from build123d import *

# Parameters (mm, degrees)
BOSS_EXTRUDE1_DEPTH       = 5.588
F_6_32_TAPPED_HOLE1_D     = 2.7051
F_6_32_TAPPED_HOLE1_DEPTH = 0.508
CUT_EXTRUDE1_REACH        = 12.16
SKETCH6_R                 = 2.159
CUT_EXTRUDE2_DEPTH        = 6.588
BOSS_EXTRUDE3_DEPTH       = 1.016
SKETCH20_W                = 9.144
SKETCH20_H                = 2.56692539
CUT_EXTRUDE3_DEPTH        = 8.382
SKETCH22_W                = 9.144
SKETCH22_H                = 8.382
BOSS_EXTRUDE4_DEPTH       = 0.508
SKETCH24_W                = 9.144
SKETCH24_H                = 8.382
BOSS_EXTRUDE5_DEPTH       = 0.508


with BuildPart() as part:
    # Sketch1 → Boss-Extrude1 (new body)
    with BuildSketch(Plane.XY):
        Polygon((-3.353873239, 7.634688699), (-3.353873239, -2.271311301), (6.806126761, -2.271311301), (6.806126761, 7.634688699), (6.298126761, 7.634688699), (6.298126761, -0.747311301), (-2.845873239, -0.747311301), (-2.845873239, 7.634688699), align=None)
    extrude(amount=BOSS_EXTRUDE1_DEPTH)

    # #6-32 Tapped Hole1
    with Locations(Plane.ZY.offset(3.353873239)):
        with Locations((2.794, 4.840688699)):
            Hole(F_6_32_TAPPED_HOLE1_D / 2, depth=F_6_32_TAPPED_HOLE1_DEPTH)

    # Sketch6 → Cut-Extrude1 (cut, up to next)
    with BuildSketch(Plane(origin=(6.806126761, 0, 0), x_dir=(0, 0, -1), z_dir=(1, 0, 0)), mode=Mode.PRIVATE) as cut_extrude1_sk1:
        with Locations((-2.794, 4.840688699)):
            Circle(SKETCH6_R)
    cut_extrude1_tool1 = extrude(cut_extrude1_sk1.sketch, amount=-CUT_EXTRUDE1_REACH, mode=Mode.PRIVATE) & part.part
    add(cut_extrude1_tool1.solids().sort_by_distance((6.806127, 4.840689, 2.794))[0], mode=Mode.SUBTRACT)

    # Sketch16 → Cut-Extrude2 (cut, through all)
    with BuildSketch(Plane(origin=(0, 0, 0), x_dir=(-1, 0, 0), z_dir=(0, 0, -1))):
        with BuildLine():
            Line((3.353873239, -2.271311301), (-6.806126761, -2.271311301))
            ThreePointArc((-6.806126761, -2.271311301), (-1.726126761, -1.350821544), (3.353873239, -2.271311301))
        make_face()
    extrude(amount=-CUT_EXTRUDE2_DEPTH, mode=Mode.SUBTRACT)

    # Sketch19 → Boss-Extrude3 (add)
    with BuildSketch(Plane.XY.offset(5.588)):
        with BuildLine():
            Line((6.806126761, 7.634688699), (6.298126761, 7.634688699))
            Line((6.298126761, 7.634688699), (-2.845873239, 7.634688699))
            Line((-2.845873239, 7.634688699), (-3.353873239, 7.634688699))
            Line((-3.353873239, 7.634688699), (-3.353873239, -2.271311301))
            ThreePointArc((-3.353873239, -2.271311301), (1.726126761, -1.350821544), (6.806126761, -2.271311301))
            Line((6.806126761, -2.271311301), (6.806126761, 7.634688699))
        make_face()
    extrude(amount=BOSS_EXTRUDE3_DEPTH)

    # Sketch20 → Cut-Extrude3 (cut)
    with BuildSketch(Plane(origin=(0, 7.634688699, 0), x_dir=(1, 0, 0), z_dir=(0, 1, 0))):
        with Locations((1.726126761, -6.871462695)):
            Rectangle(SKETCH20_W, SKETCH20_H)
    extrude(amount=-CUT_EXTRUDE3_DEPTH, mode=Mode.SUBTRACT)

    # Sketch22 → Boss-Extrude4 (add)
    with BuildSketch(Plane.XY.offset(6.604)):
        with Locations((1.726126761, 3.443688699)):
            Rectangle(SKETCH22_W, SKETCH22_H)
    extrude(amount=-BOSS_EXTRUDE4_DEPTH)

    # Sketch24 → Boss-Extrude5 (add)
    with BuildSketch(Plane(origin=(0, 0, 0), x_dir=(-1, 0, 0), z_dir=(0, 0, -1))):
        with Locations((-1.726126761, 3.443688699)):
            Rectangle(SKETCH24_W, SKETCH24_H)
    extrude(amount=-BOSS_EXTRUDE5_DEPTH)


solid = part.part
Input: part model. Units: mm. Frame: model coordinates. A direction names the side the tool comes from. Coordinates: 2 decimals unless noted, no trailing zeros. Loops run counter-clockwise (first coordinate to the right, second up) from the corner with the lowest first, then second, coordinate; pieces in that order, holes last.
Q1. Cut plane C-C (z = 5.5). Output: boundary loops of the cut face in (x, y), then the cut area to 3 significant figures.
Q2. Set-up query: faces 4 (the face through (6.298, 2.57, 3.26)), 5 (the face through (2, 3, 0)), 6 (the face through (6.556, 2.733, 3.262)). Return all of +Z, -Z, +X, -X, +Y, -Y with unobstructed straight access to the full face (end or side cutting, diameter ignored); none if empty.
Q3. Cut plane D-D (y = 5). Output: boundary loops of the cut face in (x, z).
Q4. Cut plane B-B (z = 3). Output: boundary loops of the cut face in (x, y).
Q5. Contact query for a flat-ended pin moving along its axis: pin 1 (2.5 mm diameter, centred on y = 4.84, z = 2.79, fed in from -X). Output: stop coordinate, or through.
Q6. Draft query along Z for faces 1 (the face through (1.65, -1.35, 3.26)), 2 (the face through (-2.846, 3, 3)), 3 (the face through (2, 3, 6.604)). Return one class per face: +Z half, -Z half, draft (parallel to the pull), parting line (faces both ways), or undercut.
Q7. Cut plane A-A (y = 2). Output: boundary loops of the cut face in (x, z).
Q8. Material intervals for line 1 (Z direction, x = -0.25, y = 2.75); line 2 (X direction, y = 7.25, z = 2.25); line 3 (Y direction, x = -0.5, z = 6), sorted ascending.
Working result:
1. outline: (-3.35, -2.27) arc R14.48 cw to (6.81, -2.27) - (6.81, 7.63) - (6.3, 7.63) - (6.3, -0.75) - (-2.85, -0.75) - (-2.85, 7.63) - (-3.35, 7.63) - close
1. area: 17.7 mm2
2. face 4: +Y
2. face 5: -Z, +X, -X, +Y, -Y
2. face 6: +X
3. outline: (-3.35, 0) - (6.81, 0) - (6.81, 0.64) - (6.3, 0.64) - (6.3, 0.51) - (-2.85, 0.51) - (-2.85, 1.45) - (-3.35, 1.45) - close; (-3.35, 4.14) - (-2.85, 4.14) - (-2.85, 6.1) - (6.3, 6.1) - (6.3, 4.95) - (6.81, 4.95) - (6.81, 6.6) - (-3.35, 6.6) - close
4. outline: (-3.35, -2.27) arc R14.48 cw to (6.81, -2.27) - (6.81, 2.69) - (6.3, 2.69) - (6.3, -0.75) - (-2.85, -0.75) - (-2.85, 3.5) - (-3.35, 3.5) - close; (-3.35, 6.18) - (-2.85, 6.18) - (-2.85, 7.63) - (-3.35, 7.63) - close; (6.3, 6.99) - (6.81, 6.99) - (6.81, 7.63) - (6.3, 7.63) - close
5. pin 1: passes through
6. face 1: draft
6. face 2: undercut
6. face 3: +Z half
7. outline: (-3.35, 0) - (6.81, 0) - (6.81, 6.6) - (-3.35, 6.6) - close; hole (-2.85, 0.51) - (6.3, 0.51) - (6.3, 6.1) - (-2.85, 6.1) - close
8. line 1: z = 0 to 0.51, 6.1 to 6.6
8. line 2: x = -3.35 to -2.85, 6.3 to 6.81
8. line 3: y = -1.52 to -0.75
